Autodesk Inventor part; units mm, degrees
ref_plane "YZ Plane" through (0, 0, 0) normal (1, 0, 0) x (0, 1, 0)
ref_plane "XZ Plane" through (0, 0, 0) normal (0, 1, 0) x (-1, 0, 0)
ref_plane "XY Plane" through (0, 0, 0) normal (0, 0, 1) x (1, 0, 0)
sketch "Эскиз1" plane through (0, 0, 0) normal (0, 0, 1) x (1, 0, 0)
  circle A0 centre (0, 0) radius 2.5
  line L0 (6.3509, 0) -> (3.1754, -5.5)
  line L1 (3.1754, -5.5) -> (-3.1754, -5.5)
  line L2 (-3.1754, -5.5) -> (-6.3509, 0)
  line L3 (-6.3509, 0) -> (-3.1754, 5.5)
  line L4 (-3.1754, 5.5) -> (3.1754, 5.5)
  line L5 (3.1754, 5.5) -> (6.3509, 0)
  dimension "d0" = 5
  dimension "d21" = 3
extrude "Выдавливание1" add sketch "Эскиз1" along normal blind 4
sketch "Эскиз2" plane through (0, 0, 0) normal (0, 1, 0) x (-1, 0, 0)
  line L0 (0, 0) -> (0, 12.9838)
  line L1 (-3.1754, 0) -> (-6.3509, 0) construction
  line L2 (-6.3509, 0) -> (-6.3509, 4) construction
  line L3 (-6.3509, 4) -> (-3.1754, 4) construction
  line L4 (-1.9952, -1.9581) -> (-8.8509, 2)
  line L5 (-8.8509, 2) -> (-1.9952, 5.9581)
  line L6 (-1.9952, 5.9581) -> (-9.8509, 5.9581)
  line L7 (-9.8509, 5.9581) -> (-9.8509, -1.9581)
  line L8 (-9.8509, -1.9581) -> (-1.9952, -1.9581)
  line L9 (-6.3509, 2) -> (-29.2681, 2) construction
  point P0 (-9.8509, 2)
  dimension "d4" = 60
  dimension "d5" = 1
  dimension "d6" = 3.5
revolve "Вращение1" cut sketch "Эскиз2" angle 360 about axis through (0, 0, 0) along (0, 0, 1)
sketch "Эскиз3" plane through (0, 0, 0) normal (0, 0, -1) x (-1, 0, 0)
  circle A0 centre (0, 0) radius 2.5
  circle A1 centre (0, 0) radius 5.3868
  circle A2 centre (0, 0) radius 5.3868
extrude "Выдавливание2" add sketch "Эскиз3" along normal blind 3
fillet "Сопряжение1" radius 2 1 edges at (5.3868, 0, -3)
chamfer "Фаска2" distance 0.5 angle 45 1 edges at (-2.5, 0, 4)
sketch "Sketch5" plane through (0, 0, -3) normal (0, 0, -1) x (-1, 0, 0)
  circle A0 centre (0, 0) radius 2.5
  circle A1 centre (0, 0) radius 3.3868
extrude "Extrusion4" cut sketch "Sketch5" against normal blind 0.2
fillet "Fillet3" radius 0.2 1 edges at (3.3868, 0, -3)
properties part number "paris_nut"
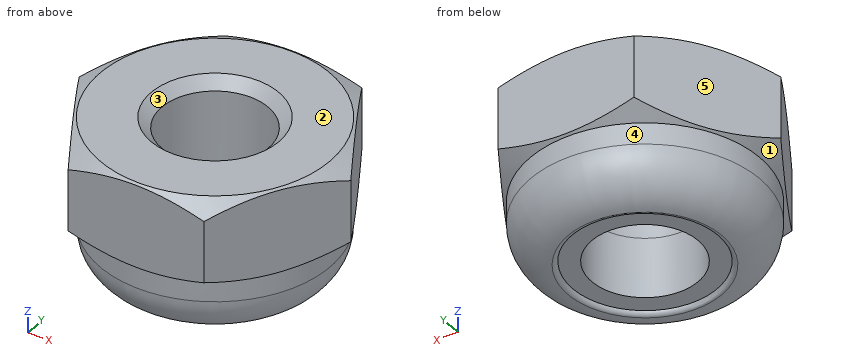
The model under review builds one solid part; all positions refer to its coordinate system, in mm. Face numbers are marked on the shaded views. A direction names the side the tool comes from. Give positions to 0.01 mm unless a question says otherwise; leave off trailing zeros. Write each loop counter-clockwise with the first axis right and the second up, starting at its lowest first coordinate (ties: lowest second). Pieces come first, ordered by that corner, then holes. Notation, with made-up numbers: M 20,56 L 63,56 A15 ccw 63,83 Z; hole C -4.5,51.5 d6. An arc over 180 degrees is marked long. One line per question, with ' | ' between items. Start each with the question number.
Item 1: Wall thickness on line 1 (Y direction, x = 0, z = 1.55); line 2 (X direction, y = 0, z = -0.7): over which ranges is each line inside the solid? List them lowest first. Write a range as from..to.
Item 2: Draft analysis for pull direction Y (two halves, no side actions). For the marked faces 1, 2 and 3, state which applies: released by +Y, released by -Y, zero draft, split by the parting line, or undercut.
Item 3: We need section C-C on z = -2. Write out the cut boundary in (x, y), plus the area to 3 significant figures.
Item 4: For the marked faces 4 and 5, list the 3-axis set-ups (+Z, -Z, +X, -X, +Y, -Y) from which the entire face can be reached by the end or side of a thin tool; tool diameter is ignored.
Item 5: We need section A-A on x = 0. Write out the cut boundary in (y, z).
Item 6: For pin 1 (2 mm diameter, centred on x = -4.5, z = 2.5, fed in from +Y); pin 2 (1.5 mm diameter, centred on y = 2, z = 2, fed in from +X), all flat-tipped, find the tip position at first contact; note any pin that passes through.
Item 7: We need section B-B on z = 1. Write out the cut boundary in (x, y), plus the area to 3 significant figures.
Item 8: We need section D-D on z = -0.5. Write out the cut boundary in (x, y).
Results found:
1) line 1: y = -5.5..-2.5, 2.5..5.5 | line 2: x = -5.39..-2.5, 2.5..5.39
2) face 1: split by the parting line | face 2: zero draft | face 3: undercut
3) outline: C 0,0 d10.24; hole C 0,0 d5 | area: 62.7 mm2
4) face 4: -Z | face 5: +Z, -Z, -X, +Y
5) outline: M -5.5,0.07 L -5.39,0 L -5.39,-1 A2 ccw -3.61,-2.99 A0.2 ccw -3.39,-2.8 L -2.5,-2.8 L -2.5,3.5 L -3,4 L -5.39,4 L -5.5,3.93 Z; M 2.5,-2.8 L 3.39,-2.8 A0.2 ccw 3.61,-2.99 A2 ccw 5.39,-1 L 5.39,0 L 5.5,0.07 L 5.5,3.93 L 5.39,4 L 3,4 L 2.5,3.5 Z
6) pin 1: stops at y = 4.94 | pin 2: stops at x = 5.63
7) outline: M -6.35,0 L -3.18,-5.5 L 3.18,-5.5 L 6.35,0 L 3.18,5.5 L -3.18,5.5 Z; hole C 0,0 d5 | area: 85.2 mm2
8) outline: C 0,0 d10.77; hole C 0,0 d5
